Could you check a few things on this model? Use its own coordinates, in mm. A direction names the side the tool comes from. Coordinates: 2 decimals unless noted, no trailing zeros. Order: outer loops, then holes, each group sorted by start corner. A loop starts at its lowest first (then second) coordinate and runs counter-clockwise, first axis right, second up.
```python
from build123d import *

# Parameters (mm, degrees)
SKETCH1_W           = 46.5
SKETCH1_H           = 50
BOSS_EXTRUDE1_DEPTH = 7
SKETCH2_W           = 33.6
SKETCH2_H           = 17.8
CUT_EXTRUDE1_DEPTH  = 2
CHAMFER1_SIZE       = 2
CUT_EXTRUDE2_DEPTH  = 4
SKETCH4_R           = 1.5
CUT_EXTRUDE3_DEPTH  = 10
SKETCH5_W           = 6
SKETCH5_H           = 7.8
CUT_EXTRUDE4_DEPTH  = 10


with BuildPart() as part:
    # Sketch1 → Boss-Extrude1 (new body)
    with BuildSketch(Plane.XY):
        Rectangle(SKETCH1_W, SKETCH1_H)
    extrude(amount=BOSS_EXTRUDE1_DEPTH)

    # Sketch2 → Cut-Extrude1 (cut)
    with BuildSketch(Plane.XY.offset(7)):
        Rectangle(SKETCH2_W, SKETCH2_H)
    extrude(amount=-CUT_EXTRUDE1_DEPTH, mode=Mode.SUBTRACT)

    # Chamfer1
    chamfer1_edges = [part.edges().sort_by_distance(p)[0] for p in [
        (0, -8.9, 5),
        (16.8, 0, 5),
        (0, 8.9, 5),
        (-16.8, 0, 5),
    ]]
    chamfer(chamfer1_edges, length=CHAMFER1_SIZE - 0.0001)  # a hair under: the kernel refuses the full size

    # Sketch3 → Cut-Extrude2 (cut)
    with BuildSketch(Plane.XY.offset(7)):
        with BuildLine():
            Line((23.25, -25), (17.25, -25))
            Line((17.25, -25), (17.25, -22))
            ThreePointArc((17.25, -22), (18.128679656, -19.878679656), (20.25, -19))
            Line((20.25, -19), (23.25, -19))
            Line((23.25, -19), (23.25, -25))
        make_face()
        with BuildLine():
            Line((-23.25, -25), (-17.25, -25))
            Line((-17.25, -25), (-17.25, -22))
            ThreePointArc((-17.25, -22), (-18.128679656, -19.878679656), (-20.25, -19))
            Line((-20.25, -19), (-23.25, -19))
            Line((-23.25, -19), (-23.25, -25))
        make_face()
        with BuildLine():
            Line((-17.25, 25), (-17.25, 22))
            ThreePointArc((-17.25, 22), (-18.128679656, 19.878679656), (-20.25, 19))
            Line((-20.25, 19), (-23.25, 19))
            Line((-23.25, 19), (-23.25, 25))
            Line((-23.25, 25), (-17.25, 25))
        make_face()
        with BuildLine():
            Line((17.25, 25), (17.25, 22))
            ThreePointArc((17.25, 22), (18.128679656, 19.878679656), (20.25, 19))
            Line((20.25, 19), (23.25, 19))
            Line((23.25, 19), (23.25, 25))
            Line((23.25, 25), (17.25, 25))
        make_face()
    extrude(amount=-CUT_EXTRUDE2_DEPTH, mode=Mode.SUBTRACT)

    # Sketch4 → Cut-Extrude3 (cut)
    with BuildSketch(Plane.XY.offset(7)):
        with Locations((-20.25, 22)):
            Circle(SKETCH4_R)
        with Locations((20.25, 22)):
            Circle(SKETCH4_R)
        with Locations((20.25, -22)):
            Circle(SKETCH4_R)
        with Locations((-20.25, -22)):
            Circle(SKETCH4_R)
    extrude(amount=-CUT_EXTRUDE3_DEPTH, mode=Mode.SUBTRACT)

    # Sketch5 → Cut-Extrude4 (cut)
    with BuildSketch(Plane.XY.offset(5)):
        with Locations((-8.8, 0)):
            Rectangle(SKETCH5_W, SKETCH5_H)
        with Locations((0.2, 0)):
            Rectangle(SKETCH5_W, SKETCH5_H)
        with Locations((9.2, 0)):
            Rectangle(SKETCH5_W, SKETCH5_H)
    extrude(amount=-CUT_EXTRUDE4_DEPTH, mode=Mode.SUBTRACT)


solid = part.part
```
Item 1: I need wall thicknesses on line 1 (Y direction, x = -20.25, z = 1); line 2 (Y direction, x = -6, z = 3.25); line 3 (Z direction, x = -8, y = 6.5). Which ranges of each line are inside material? Lowest first, please.
Item 2: Which directions (+Z, -Z, +X, -X, +Y, -Y) give clear straight access to the entire face, cutting with the end or side of a thin tool? Please do faces 1 (the face through (-17.25, -24, 5)), 2 (the face through (-22, 23, 3)), 3 (the face through (-3, 0, 5)), 4 (the face through (-2.8, 0, 3)).
Item 3: Suppose I cut it at A-A (z = 1.5). List the corners of the cut face in (x, y) for me, and give its area (3 significant figures).
Item 4: Suppose I cut it at C-C (z = 6). List the corners of the cut face in (x, y) for me.
Item 5: For pin 1 Ø1.5 at (y, z) = (-23, 6) entering from +X; pin 2 Ø5 at (x, y) = (20, -23) entering from +Z; pin 3 Ø11 at (x, y) = (7, 0.5) entering from +Z; pin 4 Ø2.5 at (x, y) = (-20.25, -22) entering from -Z, each with a flat end and sliding along its axis, tell me the tip position at first contact or that it passes through.
Item 6: Thinking about a two-plate mould opening in Y: for faces 5 (the face through (-23.25, 0, 3)), 6 (the face through (-0.2, 7.9, 6)), 7 (the face through (22, -19, 5)), 8 (the face through (22, 19, 5)), which applies, +Y half, -Y half, draft (parallel to the pull), parting line (faces both ways), or undercut?
Geometry results:
1. line 1: y = -25 to -23.5, -20.5 to 20.5, 23.5 to 25
1. line 2: y = -25 to -3.9, 3.9 to 25
1. line 3: z = 0 to 5
2. face 1: +Z, -X, -Y
2. face 2: +Z, -X, +Y
2. face 3: +Z
2. face 4: +Z, -Z
3. outline: (-23.25, -25) - (23.25, -25) - (23.25, 25) - (-23.25, 25) - close; hole circle Ø3 at (-20.25, -22); hole circle Ø3 at (-20.25, 22); hole (-11.8, -3.9) - (-5.8, -3.9) - (-5.8, 3.9) - (-11.8, 3.9) - close; hole (-2.8, -3.9) - (3.2, -3.9) - (3.2, 3.9) - (-2.8, 3.9) - close; hole (6.2, -3.9) - (12.2, -3.9) - (12.2, 3.9) - (6.2, 3.9) - close; hole circle Ø3 at (20.25, -22); hole circle Ø3 at (20.25, 22)
3. area: 2,160 mm2
4. outline: (-23.25, -19) - (-20.25, -19) arc R3 cw to (-17.25, -22) - (-17.25, -25) - (17.25, -25) - (17.25, -22) arc R3 cw to (20.25, -19) - (23.25, -19) - (23.25, 19) - (20.25, 19) arc R3 cw to (17.25, 22) - (17.25, 25) - (-17.25, 25) - (-17.25, 22) arc R3 cw to (-20.25, 19) - (-23.25, 19) - close; hole (-15.8, -7.9) - (15.8, -7.9) - (15.8, 7.9) - (-15.8, 7.9) - close
5. pin 1: stops at x = 17.25
5. pin 2: stops at z = 3
5. pin 3: stops at z = 5
5. pin 4: passes through
6. face 5: draft
6. face 6: undercut
6. face 7: -Y half
6. face 8: +Y half
